Could you check a few things on this model? Use its own coordinates, in mm. A direction names the side the tool comes from. Coordinates: 2 decimals unless noted, no trailing zeros. Write each loop counter-clockwise with the first axis right and the second up, starting at its lowest first coordinate (ties: lowest second). Pieces come first, ordered by that corner, then holes. Notation, with made-up numbers: M 35,18 L 84,18 A15 ccw 84,33 Z; hole C 3,-27.5 d7. An arc over 180 degrees is marked long. Write item = value, one per line.
```python
from build123d import *

# Parameters (mm, degrees)
F0_R     = 15
F1_DEPTH = 800
F2_R     = 50
F3_DEPTH = 10
F4_R     = 5
F5_DEPTH = 30


with BuildPart() as f1:
    # F0 (on Front) → F1 (new body)
    with BuildSketch(Plane.XZ):
        Circle(F0_R)
    extrude(amount=F1_DEPTH)

    # F2 (on face) → F3 (join)
    with BuildSketch(Plane(origin=(0, 0, 0), x_dir=(-1, 0, 0), z_dir=(0, 1, 0))):
        Circle(F2_R)
        with BuildLine():
            ThreePointArc((-17.5, -14.25), (-13.787689, -15.787689), (-12.25, -19.5))
            Line((-12.25, -19.5), (-12.25, -38))
            ThreePointArc((-12.25, -38), (-13.787689, -41.712311), (-17.5, -43.25))
            ThreePointArc((-17.5, -43.25), (-21.212311, -41.712311), (-22.75, -38))
            Line((-22.75, -38), (-22.75, -19.5))
            ThreePointArc((-22.75, -19.5), (-21.212311, -15.787689), (-17.5, -14.25))
        make_face(mode=Mode.SUBTRACT)
        with BuildLine():
            ThreePointArc((17.5, -14.25), (21.212311, -15.787689), (22.75, -19.5))
            Line((22.75, -19.5), (22.75, -38))
            ThreePointArc((22.75, -38), (21.212311, -41.712311), (17.5, -43.25))
            ThreePointArc((17.5, -43.25), (13.787689, -41.712311), (12.25, -38))
            Line((12.25, -38), (12.25, -19.5))
            ThreePointArc((12.25, -19.5), (13.787689, -15.787689), (17.5, -14.25))
        make_face(mode=Mode.SUBTRACT)
        with BuildLine():
            Line((-22.75, 19.5), (-22.75, 38))
            ThreePointArc((-22.75, 38), (-21.212311, 41.712311), (-17.5, 43.25))
            ThreePointArc((-17.5, 43.25), (-13.787689, 41.712311), (-12.25, 38))
            Line((-12.25, 38), (-12.25, 19.5))
            ThreePointArc((-12.25, 19.5), (-13.787689, 15.787689), (-17.5, 14.25))
            ThreePointArc((-17.5, 14.25), (-21.212311, 15.787689), (-22.75, 19.5))
        make_face(mode=Mode.SUBTRACT)
        with BuildLine():
            ThreePointArc((17.5, 43.25), (21.212311, 41.712311), (22.75, 38))
            Line((22.75, 38), (22.75, 19.5))
            ThreePointArc((22.75, 19.5), (21.212311, 15.787689), (17.5, 14.25))
            ThreePointArc((17.5, 14.25), (13.787689, 15.787689), (12.25, 19.5))
            Line((12.25, 19.5), (12.25, 38))
            ThreePointArc((12.25, 38), (13.787689, 41.712311), (17.5, 43.25))
        make_face(mode=Mode.SUBTRACT)
    extrude(amount=F3_DEPTH)

    # F4 (on face) → F5 (cut)
    with BuildSketch(Plane.XZ.offset(800)):
        Circle(F4_R)
    extrude(amount=-F5_DEPTH, mode=Mode.SUBTRACT)


solid = f1.part
```
Item 1: If I drill on line 1 along Z through (x, y) = (0, -781); line 2 along X through (y, z) = (-440, 4.5); line 3 along Z through (x, y) = (-5, -717.5), over which ranges is the centre line in solid material (lowest first)?
Numbers:
line_1 = -15 to -5, 5 to 15
line_2 = -14.31 to 14.31
line_3 = -14.14 to 14.14
Item 2: For faces 1 (the face through (-47.69, 4.93, 15.02)), 2 (the face through (-14.985, -394.4, 0.66)), which set-ups out of +Z, -Z, +X, -X, +Y, -Y let a thin tool reach every point of the face, with its end or its side?
Numbers:
face_1 = +Y, -Y
face_2 = -Y
Item 3: Imagine slicing it at B-B (x = -29.5). Write out the boundary of the cut face in (y, z).
Numbers:
outline = M 0,-40.37 L 10,-40.37 L 10,40.37 L 0,40.37 Z
Item 4: I'm going to push flat-ended pins straight in: P1, Ø11, axis at y = 7.5, z = -32, coming from the +X side; P2, Ø11, axis at y = 4, z = 29.5, coming from the -X side; P3, Ø11, axis at y = 3, z = -25, coming from the -X side. Where does each tip first touch, or does it pass through?
Numbers:
P1 = 42.4
P2 = -43.86
P3 = -46.04
Item 5: Imagine slicing it at A-A (y = -671.5). Write out the boundary of the cut face in (x, z), and give its area (3 significant figures).
Numbers:
outline = C 0,0 d30
area = 707 mm²
